Autodesk Inventor part; units mm, degrees
ref_plane "Work Plane2" through (-8.2623, 8.1273, 0) normal (0, 1, 0) x (1, 0, 0)
ref_plane "YZ Plane" through (0, 0, 0) normal (1, 0, 0) x (0, 1, 0)
ref_plane "XZ Plane" through (0, 0, 0) normal (0, 1, 0) x (-1, 0, 0)
ref_plane "Work Plane6" through (0, 0, 31.75) normal (0, 0, 1) x (1, 0, 0)
sketch "Sketch4" plane through (0, 0, 31.75) normal (0, 0, 1) x (1, 0, 0)
  line L0 (17.1377, 8.1273) -> (-8.2623, 8.1273)
  line L1 (4.4377, 8.1273) -> (4.4377, -17.2727)
  line L2 (-8.2623, -17.2727) -> (17.1377, -17.2727)
  circle A0 centre (4.4377, -4.5727) radius 25.4
  point P0 (0, 0)
  dimension "d11" = 50.8
extrude "Extrusion4" add sketch "Sketch4" along normal blind 101.6
ref_plane "Work Plane2" through (-8.2623, 8.1273, 0) normal (0, 1, 0) x (1, 0, 0)
sketch "Sketch5" plane through (-8.2623, 8.1273, 0) normal (0, 1, 0) x (1, 0, 0)
  line L0 (25.4, 0) -> (0, 0)
  line L1 (-12.7, -133.35) -> (38.1, -133.35)
  circle A0 centre (12.7, -111.125) radius 9.525
  point P0 (8.2623, 0)
extrude "Extrusion5" cut sketch "Sketch5" along normal blind 101.6
sketch "Sketch6" plane through (4.4377, 8.1273, 111.125) normal (0, 1, 0) x (1, 0, 0)
  circle A0 centre (0, 0) radius 9.525
  point P0 (-4.4377, 111.125)
extrude "Extrusion6" cut sketch "Sketch6" against normal blind 6.35
sketch "Sketch13" plane through (4.4377, -4.5727, 31.75) normal (0, 0, -1) x (-1, 0, 0)
  circle A0 centre (0, 0) radius 38.1
  point P0 (4.4377, 4.5727)
  dimension "d36" = 76.2
extrude "Extrusion11" add sketch "Sketch13" along normal blind 12.7
sketch "Sketch14" plane through (4.4377, -4.5727, 133.35) normal (0, 0, 1) x (1, 0, 0)
  circle A0 centre (0, 0) radius 19.05
  circle A1 centre (0, 0) radius 25.4
  point P0 (-4.4377, 4.5727)
  dimension "d39" = 38.1
extrude "Extrusion12" cut sketch "Sketch14" against normal blind 101.6
sketch "Sketch15" plane through (4.4377, -4.5727, 31.75) normal (0, 0, 1) x (1, 0, 0)
  circle A0 centre (0, 0) radius 19.05
  line L0 (-19.05, 0) -> (-38.1, 0)
  circle A1 centre (0, 0) radius 38.1
  line L1 (0, 38.1) -> (0, 19.0375)
  line L2 (19.05, 0) -> (38.1, 0)
  line L3 (0, -19.05) -> (0, -38.1)
  circle A2 centre (-28.575, 0) radius 1.5875
  circle A3 centre (28.575, 0) radius 1.5875
  circle A4 centre (0, 28.5687) radius 1.5875
  circle A5 centre (0, -28.575) radius 1.5875
  point P0 (-4.4377, 4.5727)
  dimension "d42" = 3.175
  dimension "d43" = 3.175
  dimension "d44" = 3.175
  dimension "d45" = 3.175
extrude "Extrusion13" cut sketch "Sketch15" against normal blind 101.6 contours A2 L0 | L0 A2 | A5 L3 | L3 A5 | A4 L1 | L1 A4 | A3 L2 | L2 A3
properties part number "CrankP1_SBail"
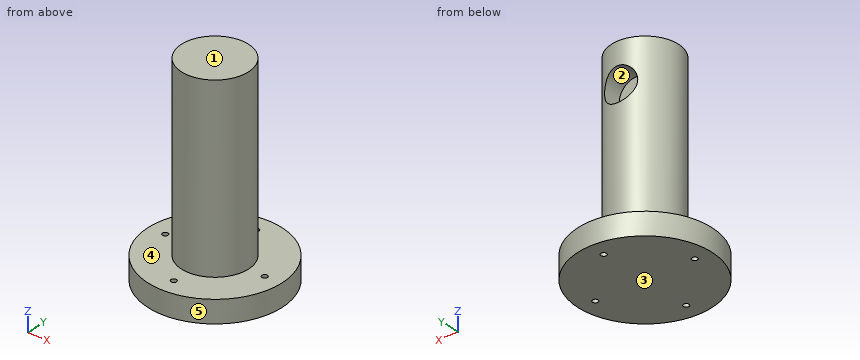
Geometry check sheet. Reference: the model listing, model coordinates, mm. Face numbers are marked on the shaded views. A direction names the side the tool comes from. Round coordinates to 2 decimals unless told otherwise and drop trailing zeros. Write each loop counter-clockwise with the first axis right and the second up, starting at its lowest first coordinate (ties: lowest second). Pieces come first, ordered by that corner, then holes. Notation, with made-up numbers: (15.25, -29.75) -> (60.25, -29.75) arc R29 cw to (60.25, 0.25) -> close; hole circle Ø5 at (-10, 17.5). An arc over 180 degrees is marked (long way). One line per item, written item: value. Start each with the question number.
(1) Scan lines: line 1 (Z direction, x = 4, y = 13.5); line 2 (Z direction, x = 8, y = 18.5); line 3 (Z direction, x = -4, y = 10). Record each from-to range of solid material in increasing order. Write a range as [from, to].
(2) Go/stop test with flat-tipped pins: pin 1 Ø11.5 at (x, z) = (4.44, 111.12) entering from +Y; pin 2 Ø1 at (x, z) = (20.5, 68.5) entering from +Y; pin 3 Ø10 at (y, z) = (-24.5, 35) entering from +X. Record where each tip stops, or that it passes through.
(3) Cross-section at C-C, the plane z = 29. Record the cut outline in (x, y) (1 decimal), and give its area (3 significant figures).
(4) Cross-section at A-A, the plane x = 15.5. Record the cut outline in (y, z).
(5) Cross-section at B-B, the plane y = 6. Record the cut outline in (x, z) (3 decimals), and give its area (3 significant figures).
(6) Access from +Z, -Z, +X, -X, +Y, -Y to the whole of each face (thin tool, end or side, straight path). Record for the marked faces 4 and 5.
(7) Cross-section at D-D, the plane y = -12. Record the cut outline in (x, z), and give its area (3 significant figures).
(8) Draft check along Z on the marked faces 1, 2 and 3. Enter one of: +Z half, -Z half, draft (parallel to the pull), parting line (faces both ways), or undercut.
Answer:
1. line 1: [19.05, 101.61], [120.64, 133.35]
1. line 2: [19.05, 31.75]
1. line 3: [19.05, 106.71], [115.54, 133.35]
2. pin 1: y = 1.78
2. pin 2: y = 6.41
2. pin 3: x = 38.96
3. outline: circle Ø76.2 at (4.4, -4.6); hole circle Ø3.2 at (-24.1, -4.6); hole circle Ø3.2 at (4.4, -33.1); hole circle Ø3.2 at (4.4, 24); hole circle Ø3.2 at (33, -4.6)
3. area: 4,530 mm²
4. outline: (-41.03, 19.05) -> (31.89, 19.05) -> (31.89, 31.75) -> (10.94, 31.75) -> (10.94, 133.35) -> (-20.08, 133.35) -> (-20.08, 31.75) -> (-41.03, 31.75) -> close
5. outline: (-32.166, 19.05) -> (41.041, 19.05) -> (41.041, 31.75) -> (20.284, 31.75) -> (20.284, 133.35) -> (-11.409, 133.35) -> (-11.409, 31.75) -> (-32.166, 31.75) -> close; hole circle Ø19.05 at (4.438, 111.125)
5. area: 3,860 mm²
6. face 4: +Z
6. face 5: +Z, -Z
7. outline: (-32.93, 19.05) -> (41.81, 19.05) -> (41.81, 31.75) -> (21.98, 31.75) -> (21.98, 133.35) -> (-13.1, 133.35) -> (-13.1, 31.75) -> (-32.93, 31.75) -> close
7. area: 4,510 mm²
8. face 1: +Z half
8. face 2: undercut
8. face 3: -Z half
